Here's how the part is built. I have some questions about the finished solid (model axes, mm). Give positions to 0.01 mm unless a question says otherwise; leave off trailing zeros. Order: outer loops, then holes, each group sorted by start corner. A loop starts at its lowest first (then second) coordinate and runs counter-clockwise, first axis right, second up.
from build123d import *

# Parameters (mm, degrees)
SKETCH_1_W      = 232
SKETCH_1_H      = 31
SKETCH_1_R      = 2.25
EXTRUDE_1_DEPTH = 2


with BuildPart() as part:
    # Эскиз1 → Вытянуть1 (new body)
    with BuildSketch(Plane.XY):
        Rectangle(SKETCH_1_W, SKETCH_1_H)
        with Locations((-28, 7)):
            Circle(SKETCH_1_R, mode=Mode.SUBTRACT)
        with Locations((28, 7)):
            Circle(SKETCH_1_R, mode=Mode.SUBTRACT)
        with Locations((-94, 7)):
            Circle(SKETCH_1_R, mode=Mode.SUBTRACT)
        with Locations(Location((94, 7, 0), (0, 0, 180))):
            Circle(SKETCH_1_R, mode=Mode.SUBTRACT)
        with Locations((-107, -10.5)):
            Circle(SKETCH_1_R, mode=Mode.SUBTRACT)
        with Locations((107, -10.5)):
            Circle(SKETCH_1_R, mode=Mode.SUBTRACT)
    extrude(amount=EXTRUDE_1_DEPTH)


solid = part.part
Q1. I'm going to push flat-ended pins straight in: P1, Ø5, axis at x = 23.5, y = 9.5, coming from the -Z side; P2, Ø2.5, axis at x = 94, y = 7, coming from the -Z side. Where does each tip first touch, or does it pass through?
Filled sheet:
P1: stops at z = 0
P2: passes through
Q2. Thinking about a two-plate mould opening in X: for faces 1 (the face through (-2, 0, 0)), 2 (the face through (-91.854, 7.676, 0.986)), which applies, released by +X, released by -X, zero draft, split by the parting line, or undercut?
Filled sheet:
face 1: zero draft
face 2: undercut
Q3. If we section it at A-A on x = -94: List the corners of the cut face in (y, z) for me, plus the area to 3 significant figures.
Filled sheet:
outline: (-15.5, 0) - (4.75, 0) - (4.75, 2) - (-15.5, 2) - close; (9.25, 0) - (15.5, 0) - (15.5, 2) - (9.25, 2) - close
area: 53.0 mm2
Q4. I need wall thicknesses on L1, parallel to Y at x = 28, z = 1.55; L2, parallel to Y at x = -107, z = 0.8; L3, parallel to X at y = 8.5, z = 0.6. Which ranges of each line are inside material? Lowest first, please.
Filled sheet:
L1: y = -15.5 to 4.75, 9.25 to 15.5
L2: y = -15.5 to -12.75, -8.25 to 15.5
L3: x = -116 to -95.68, -92.32 to -29.68, -26.32 to 26.32, 29.68 to 92.32, 95.68 to 116
Q5. If we section it at B-B on y = 7: List the corners of the cut face in (x, z) for me, plus the area to 3 significant figures.
Filled sheet:
outline: (-116, 0) - (-96.25, 0) - (-96.25, 2) - (-116, 2) - close; (-91.75, 0) - (-30.25, 0) - (-30.25, 2) - (-91.75, 2) - close; (-25.75, 0) - (25.75, 0) - (25.75, 2) - (-25.75, 2) - close; (30.25, 0) - (91.75, 0) - (91.75, 2) - (30.25, 2) - close; (96.25, 0) - (116, 0) - (116, 2) - (96.25, 2) - close
area: 428 mm2
